```python
from build123d import *

# Parameters (mm, degrees)
BOSS_EXTRUDE1_DEPTH = 4
CHAMFER1_SIZE       = 0.2
CHAMFER1_SIZE_2     = 0.206341937
CHAMFER2_SIZE       = 0.5


with BuildPart() as part:
    # Sketch1 → Boss-Extrude1 (new body)
    with BuildSketch(Plane(origin=(0, 0, 0), x_dir=(1, 0, 0), z_dir=(0, 1, 0))):
        with BuildLine():
            ThreePointArc((5, 0), (1.227434059, 4.846999652), (-4.397362252, 2.379748983))
            Line((-4.397362252, 2.379748983), (-2.883140649, 1.5))
            ThreePointArc((-2.883140649, 1.5), (0.772105204, 3.156953207), (3.25, 0))
            ThreePointArc((3.25, 0), (0.772105204, -3.156953207), (-2.883140649, -1.5))
            Line((-2.883140649, -1.5), (-4.397362252, -2.379748983))
            ThreePointArc((-4.397362252, -2.379748983), (1.227434059, -4.846999652), (5, 0))
        make_face()
    extrude(amount=BOSS_EXTRUDE1_DEPTH)

    # Chamfer1
    # the kernel refuses this chamfer: 0.206341937, 0.2, 0.191297121 mm, written as the material it takes off along each edge
    with BuildSketch(Plane(origin=(-2.883140649, -0.514336598, -1.5), x_dir=(0.4881882615859918, 0, -0.8727383463843256), z_dir=(0, 1, 0))) as chamfer1_piece_1:
        with BuildLine():
            Line((0.196815803, 0), (CHAMFER1_SIZE * 0.0163116056584, CHAMFER1_SIZE * 0.99986695691))
            Line((CHAMFER1_SIZE * 0.0163116056584, CHAMFER1_SIZE * 0.99986695691), (0, 0))
            ThreePointArc((0, 0), (0.101193556, 0.001489012), (0.196815803, 0))
        make_face()
    extrude(amount=5.028673195, mode=Mode.SUBTRACT)
    with BuildSketch(Plane(origin=(-4.397362252, -0.531068819, -2.379748983), x_dir=(0.4931124519861111, 0, -0.8699655796042999), z_dir=(0, 1, 0))) as chamfer1_piece_2:
        with BuildLine():
            Line((0.196188757, 0), (-CHAMFER1_SIZE_2 * 0.010660935079, -CHAMFER1_SIZE_2 * 0.999943172174))
            Line((-CHAMFER1_SIZE_2 * 0.010660935079, -CHAMFER1_SIZE_2 * 0.999943172174), (0, 0))
            ThreePointArc((0, 0), (0.100953531, 0.000961526), (0.196188757, 0))
        make_face()
    extrude(amount=5.062137639, mode=Mode.SUBTRACT)
    with BuildSketch(Plane(origin=(-4.397362252, -0.520052168, 2.379748983), x_dir=(0.49362201920020077, 0, 0.8696765503109283), z_dir=(0, 1, 0))) as chamfer1_piece_3:
        with BuildLine():
            Line((0.202045895, 0), (-CHAMFER1_SIZE * 0.0100751366451, CHAMFER1_SIZE * 0.999949244523))
            Line((-CHAMFER1_SIZE * 0.0100751366451, CHAMFER1_SIZE * 0.999949244523), (0, 0))
            ThreePointArc((0, 0), (0.103969214, -0.0010198), (0.202045895, 0))
        make_face()
    extrude(amount=5.040104337, mode=Mode.SUBTRACT)
    # the kernel refuses this chamfer: 0.206341937, 0.2, 0.191297121 mm, written as the material it takes off along each edge
    with BuildSketch(Plane(origin=(-2.438414829, 4, 1.241618342), x_dir=(0.502359075260422, 0, 0.8646591001680913), z_dir=(-0.8646591001680914, 0, 0.502359075260422))) as chamfer1_2_piece_1:
        Polygon((CHAMFER1_SIZE, 0), (0, -CHAMFER1_SIZE), (0, 0), align=None)
    extrude(amount=2.57990857, mode=Mode.SUBTRACT)

    # Chamfer2
    # the kernel refuses this chamfer: 0.5 mm, written as the material it takes off along each edge
    with BuildSketch(Plane(origin=(0, 4, 0), x_dir=(-0.9618869269385497, 0, -0.2734475082803154), z_dir=(-0.2734475082803154, 0, 0.9618869269385497))) as chamfer2_piece_1:
        Polygon((5, CHAMFER2_SIZE), (5 - CHAMFER2_SIZE, 0), (5, 0), align=None)
    revolve(axis=Axis((0, 4, 0), (0, -1, 0)), revolution_arc=328.193834559, mode=Mode.SUBTRACT)


solid = part.part
```
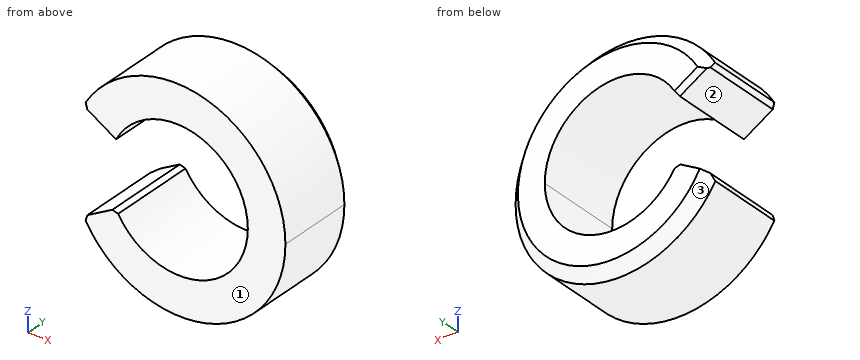
Model file for the job. Use its own axes, mm. Face numbers are marked on the shaded views. Round coordinates to 2 decimals unless told otherwise and drop trailing zeros. Order: outer loops, then holes, each group sorted by start corner. A loop starts at its lowest first (then second) coordinate and runs counter-clockwise, first axis right, second up. Notation, with made-up numbers: M 48,89 L 57,89 A29 ccw 57,119 Z; hole C 55.25,7.25 d2. An arc over 180 degrees is marked long. Use CSV: the item, a comma, the result in double quotes.
Item 1: Probe probe 1 along Z at (x, y) = (0.5, 3.35); probe 2 along Z at (x, y) = (-3.5, 2.7); probe 3 along X at (y, z) = (0.25, 0.75). List the from-to ranges inside material, lowest first.
Worked answers:
probe 1,"-4.97 to -3.21, 3.21 to 4.97"
probe 2,"-3.57 to -1.86, 1.86 to 3.57"
probe 3,"3.16 to 4.94"
Item 2: Pin check, flat tips, straight feed: pin 1 (1 mm diameter, centred on x = -2, y = 2.5, fed in from +Z); pin 2 (2 mm diameter, centred on x = -2.5, y = 3.5, fed in from -Z); pin 3 (1.5 mm diameter, centred on x = 2.5, z = -1, fed in from -Y); pin 4 (2 mm diameter, centred on y = 3, z = 2, fed in from -X). Stop position of each tip, or through.
Worked answers:
pin 1,"z = 4.77"
pin 2,"z = -4.77"
pin 3,"y = 0"
pin 4,"x = -4.3"
Item 3: Pull direction X, two halves, no side cores. Call the marked faces 1, 2 and 3: released by +X, released by -X, zero draft, split by the parting line, or undercut.
Worked answers:
face 1,"zero draft"
face 2,"released by -X"
face 3,"split by the parting line"
Item 4: Saw through at A-A (x = 0). List the corners of the cut face in (y, z).
Worked answers:
outline,"M 0,-5 L 3.5,-5 L 4,-4.5 L 4,-3.25 L 0,-3.25 Z; M 0,3.25 L 4,3.25 L 4,4.5 L 3.5,5 L 0,5 Z"
Item 5: Saw through at B-B (y = 2.6). List the corners of the cut face in (x, z).
Worked answers:
outline,"M -4.3,-2.55 A5 ccw long -4.3,2.56 L -4.22,2.28 L -2.88,1.5 A3.25 cw long -2.79,-1.67 L -3.06,-1.6 L -4.22,-2.28 Z"
